Part print with two shaded views. Sizes in mm from the minimum x, y, z corner. A direction names the side the tool comes from. Round coordinates to 2 decimals unless told otherwise and drop trailing zeros. Order: outer loops, then holes, each group sorted by start corner. A loop starts at its lowest first (then second) coordinate and runs counter-clockwise, first axis right, second up. Notation, with made-up numbers: (79.25, 74.5) -> (105.25, 74.5) arc R17 ccw to (105.25, 93.5) -> close; hole circle Ø11 at (29, 87). An arc over 180 degrees is marked (long way). Put each result on its own line as item: value. Start each with the question number.
Q1. Cut at C-C, the plane z = 127. List the corners of the cut face in (x, y), and give its area (3 significant figures).
Q2. Probe L1, parallel to Z at x = 15.5, y = 31.75 (1 decimal); L2, parallel to Z at x = 40, y = 31 (1 decimal); L3, parallel to X at y = 31, z = 33.5. List the from-to ranges inside material, lowest first.
Q3. Cut at A-A, the plane y = 31.75. State how many separate pieces and enclosed holes the cut face has, and give its area (3 significant figures).
Q4. 3-axis set-ups, long thin cutter, end or side, ignore diameter. For the marked faces 1 and 2: which of +Z, -Z, +X, -X, +Y, -Y reach the whole face in a straight line?
Q5. Flat gauge pins, fed straight in: P1, Ø18.5, axis at y = 31.75, z = 396.875, coming from the -X side; P2, Ø6, axis at y = 49, z = 49, coming from the +X side; P3, Ø12, axis at y = 24.5, z = 117.5, coming from the +X side; P4, Ø14.5, axis at y = 31.75, z = 396.875, coming from the -X side. Where does each tip first touch, or does it go through?
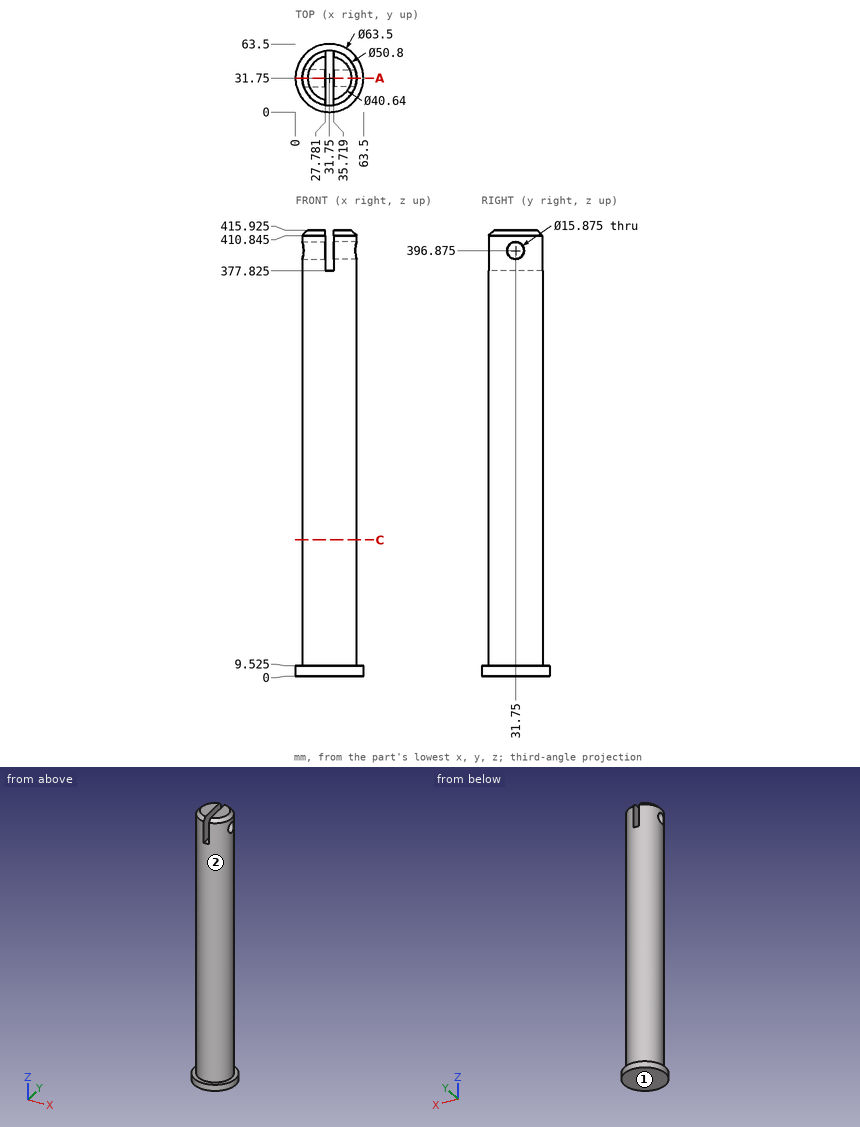
Ans:
1. outline: circle Ø50.8 at (31.75, 31.75)
1. area: 2,030 mm^2
2. L1: z = 0 to 388.9, 404.8 to 415.9
2. L2: z = 0 to 389, 404.8 to 415.9
2. L3: x = 6.36 to 57.14
3. separate pieces: 3
3. enclosed holes: 0
3. area: 20,200 mm^2
4. face 1: -Z, +X, -X, +Y, -Y
4. face 2: +Z
5. P1: stops at x = 6.35
5. P2: stops at x = 52.78
5. P3: stops at x = 57.12
5. P4: passes through
